```python
from build123d import *

# Parameters (mm, degrees)
SKETCH1_W                 = 77.5
SKETCH1_H                 = 31.5
BOSS_EXTRUDE1_DEPTH       = 2
CUT_EXTRUDE1_DEPTH        = 42.87630595
CUT_EXTRUDE1_DEPTH_BACK   = 42.87630595
SKETCH2_R                 = 1.75
CUT_EXTRUDE2_DEPTH        = 42.87630595
CUT_EXTRUDE2_DEPTH_BACK   = 42.87630595
SKETCH3_W                 = 8.5
SKETCH3_H                 = 15
BOSS_EXTRUDE2_START       = 3
SKETCH4_R                 = 2.5
SKETCH4_R_2               = 1.75
BOSS_EXTRUDE2_DEPTH       = 3
MIRROR2_START             = 3
MIRROR2_COPY_1_SKETCH_R   = 2.5
MIRROR2_COPY_1_SKETCH_R_2 = 1.75
MIRROR2_COPY_1_DEPTH      = 3
CUT_EXTRUDE3_DEPTH        = 3.5
SKETCH6_W                 = 8
SKETCH6_H                 = 10
SKETCH6_W_2               = 5
SKETCH6_H_2               = 4
BOSS_EXTRUDE3_DEPTH       = 3
SKETCH7_W                 = 16
SKETCH7_H                 = 7.5
BOSS_EXTRUDE4_DEPTH       = 3
CUT_EXTRUDE4_DEPTH        = 1
FILLET1_R                 = 10
FILLET2_R                 = 10
SKETCH9_R                 = 4
BOSS_EXTRUDE6_DEPTH       = 1.5


with BuildPart() as part:
    # Sketch1 → Boss-Extrude1 (new body)
    with BuildSketch(Plane(origin=(0, 0, 0), x_dir=(1, 0, 0), z_dir=(0, 1, 0))):
        Rectangle(SKETCH1_W, SKETCH1_H)
    extrude(amount=BOSS_EXTRUDE1_DEPTH)

    # Sketch2 → Cut-Extrude1 (cut, two sides: drawn at the far end of the back side and taken through both)
    with BuildSketch(Plane(origin=(0, 2, 0), x_dir=(1, 0, 0), z_dir=(0, 1, 0)).offset(-CUT_EXTRUDE1_DEPTH_BACK)):
        with Locations(Location((-35.75, 12.5, 0), (0, 0, 270))):
            Circle(SKETCH2_R)
        with Locations(Location((-35.75, -12.5, 0), (0, 0, 270))):
            Circle(SKETCH2_R)
        with Locations(Location((35.75, -12.5, 0), (0, 0, 270))):
            Circle(SKETCH2_R)
        with Locations(Location((35.75, 12.5, 0), (0, 0, 270))):
            Circle(SKETCH2_R)
    extrude(amount=CUT_EXTRUDE1_DEPTH + CUT_EXTRUDE1_DEPTH_BACK, mode=Mode.SUBTRACT)

    # Sketch3 → Cut-Extrude2 (cut, two sides: drawn at the far end of the back side and taken through both)
    with BuildSketch(Plane(origin=(0, 2, 0), x_dir=(1, 0, 0), z_dir=(0, 1, 0)).offset(-CUT_EXTRUDE2_DEPTH_BACK)):
        with Locations((31.5, 0)):
            Rectangle(SKETCH3_W, SKETCH3_H)
        with Locations((-31.5, 0)):
            Rectangle(SKETCH3_W, SKETCH3_H)
    extrude(amount=CUT_EXTRUDE2_DEPTH + CUT_EXTRUDE2_DEPTH_BACK, mode=Mode.SUBTRACT)

    # Sketch4 → Boss-Extrude2 (add)
    with BuildSketch(Plane(origin=(0, 2, 0), x_dir=(1, 0, 0), z_dir=(0, 1, 0)).offset(BOSS_EXTRUDE2_START)):
        with Locations(Location((-35.75, 12.5, 0), (0, 0, 270))):
            Circle(SKETCH4_R)
        with Locations(Location((-35.75, 12.5, 0), (0, 0, 270))):
            Circle(SKETCH4_R_2, mode=Mode.SUBTRACT)
    boss_extrude2 = extrude(amount=-BOSS_EXTRUDE2_DEPTH)

    # Mirror1: Boss-Extrude2 across plane
    add(boss_extrude2.mirror(Plane.XY))

    # Mirror2: Boss-Extrude2 across plane
    add(boss_extrude2.mirror(Plane(origin=(0, 0, 0), x_dir=(0, 0, 1), z_dir=(1, 0, 0))))

    # Mirror2 copy 1 sketch → Mirror2 copy 1 (add)
    with BuildSketch(Plane(origin=(0, 2, 0), x_dir=(-1, 0, 0), z_dir=(0, 1, 0)).offset(MIRROR2_START)):
        with Locations(Location((-35.75, 12.5, 0), (0, 0, 270))):
            Circle(MIRROR2_COPY_1_SKETCH_R)
        with Locations(Location((-35.75, 12.5, 0), (0, 0, 270))):
            Circle(MIRROR2_COPY_1_SKETCH_R_2, mode=Mode.SUBTRACT)
    extrude(amount=-MIRROR2_COPY_1_DEPTH)

    # Sketch5 → Cut-Extrude3 (cut)
    with BuildSketch(Plane(origin=(0, 2, 0), x_dir=(1, 0, 0), z_dir=(0, 1, 0))):
        with BuildLine():
            Line((19.75, -4.75), (19.75, 3.25))
            Line((19.75, 3.25), (20.25, 3.25))
            Line((20.25, 3.25), (20.25, -4.75))
            ThreePointArc((20.25, -4.75), (14.75, -10.25), (9.25, -4.75))
            Line((9.25, -4.75), (9.25, 3.25))
            Line((9.25, 3.25), (9.75, 3.25))
            Line((9.75, 3.25), (9.75, -4.75))
            ThreePointArc((9.75, -4.75), (14.75, -9.75), (19.75, -4.75))
        make_face()
        with BuildLine():
            Line((-19.75, 3.25), (-20.25, 3.25))
            Line((-20.25, 3.25), (-20.25, -4.75))
            ThreePointArc((-20.25, -4.75), (-14.75, -10.25), (-9.25, -4.75))
            Line((-9.25, -4.75), (-9.25, 3.25))
            Line((-9.25, 3.25), (-9.75, 3.25))
            Line((-9.75, 3.25), (-9.75, -4.75))
            ThreePointArc((-9.75, -4.75), (-14.75, -9.75), (-19.75, -4.75))
            Line((-19.75, -4.75), (-19.75, 3.25))
        make_face()
    extrude(amount=-CUT_EXTRUDE3_DEPTH, mode=Mode.SUBTRACT)

    # Sketch6 → Boss-Extrude3 (add)
    with BuildSketch(Plane(origin=(0, 2, 0), x_dir=(1, 0, 0), z_dir=(0, 1, 0))):
        with Locations((0, -2.75)):
            Rectangle(SKETCH6_W, SKETCH6_H)
        with Locations((5.5, 11.75)):
            Rectangle(SKETCH6_W_2, SKETCH6_H_2)
        with Locations((17.5, 11.75)):
            Rectangle(SKETCH6_W_2, SKETCH6_H_2)
        with Locations((-17.5, 11.75)):
            Rectangle(SKETCH6_W_2, SKETCH6_H_2)
        with Locations((-5.5, 11.75)):
            Rectangle(SKETCH6_W_2, SKETCH6_H_2)
    extrude(amount=BOSS_EXTRUDE3_DEPTH)

    # Sketch7 → Boss-Extrude4 (add)
    with BuildSketch(Plane(origin=(0, 2, 0), x_dir=(1, 0, 0), z_dir=(0, 1, 0))):
        with Locations((0, 6)):
            Rectangle(SKETCH7_W, SKETCH7_H)
    extrude(amount=BOSS_EXTRUDE4_DEPTH)

    # Sketch8 → Cut-Extrude4 (cut)
    with BuildSketch(Plane(origin=(0, 2, 0), x_dir=(1, 0, 0), z_dir=(0, 1, 0))):
        with BuildLine():
            Line((-9.75, 3.25), (-9.75, -4.75))
            ThreePointArc((-9.75, -4.75), (-14.75, -9.75), (-19.75, -4.75))
            Line((-19.75, -4.75), (-19.75, 3.25))
            Line((-19.75, 3.25), (-9.75, 3.25))
        make_face()
        with BuildLine():
            Line((19.75, 3.25), (9.75, 3.25))
            Line((9.75, 3.25), (9.75, -4.75))
            ThreePointArc((9.75, -4.75), (14.75, -9.75), (19.75, -4.75))
            Line((19.75, -4.75), (19.75, 3.25))
        make_face()
    extrude(amount=-CUT_EXTRUDE4_DEPTH, mode=Mode.SUBTRACT)

    # Fillet1
    # the kernel refuses this fillet: 10 mm, written as the material it takes off along each edge
    with BuildSketch(Plane(origin=(-4.75, 2, -3.25), x_dir=(0, 0, -1), z_dir=(-1, 0, 0))) as fillet1_piece_1_section:
        with BuildLine():
            CenterArc((6, 10), FILLET1_R, 233.130102354, 36.869897646)
            Line((0, 2), (0, 0))
            Line((0, 0), (6, 0))
        make_face()
    fillet1_piece_1 = extrude(amount=15.5, mode=Mode.PRIVATE)
    fillet1_piece_1 = split(fillet1_piece_1, bisect_by=Plane(origin=(-9.25, 2, -3.25), z_dir=(-1, 0, 0)), keep=Keep.TOP, mode=Mode.PRIVATE)
    fillet1_piece_1 = split(fillet1_piece_1, bisect_by=Plane(origin=(-4.75, 1, -3.25), z_dir=(0, 1, 0)), keep=Keep.TOP, mode=Mode.PRIVATE)
    add(fillet1_piece_1, mode=Mode.SUBTRACT)
    with BuildSketch(Plane(origin=(-4.75, 2, -3.25), x_dir=(0, 0, -1), z_dir=(-1, 0, 0))) as fillet1_piece_2_section:
        with BuildLine():
            CenterArc((6, 10), FILLET1_R, 233.130102354, 36.869897646)
            Line((0, 2), (0, 0))
            Line((0, 0), (6, 0))
        make_face()
    fillet1_piece_2 = extrude(amount=30.5, mode=Mode.PRIVATE)
    fillet1_piece_2 = split(fillet1_piece_2, bisect_by=Plane(origin=(-9.25, 2, -3.25), z_dir=(-1, 0, 0)), keep=Keep.TOP, mode=Mode.PRIVATE)
    fillet1_piece_2 = split(fillet1_piece_2, bisect_by=Plane(origin=(-9.75, 2, -3.25), z_dir=(1, 0, 0)), keep=Keep.TOP, mode=Mode.PRIVATE)
    add(fillet1_piece_2, mode=Mode.SUBTRACT)
    with BuildSketch(Plane(origin=(-19.75, 2, -3.25), x_dir=(0, 0, -1), z_dir=(-1, 0, 0)), Plane(origin=(-9.25, 2, -3.25), x_dir=(0, 0, -1), z_dir=(-1, 0, 0))) as fillet1_piece_3:
        with BuildLine():
            CenterArc((6, 10), FILLET1_R, 233.130102354, 36.869897646)
            Line((0, 2), (0, 0))
            Line((0, 0), (6, 0))
        make_face()
    extrude(amount=0.5, mode=Mode.SUBTRACT)
    with BuildSketch(Plane(origin=(-9.25, 2, -3.25), x_dir=(0, 0, -1), z_dir=(-1, 0, 0))) as fillet1_piece_4_section:
        with BuildLine():
            CenterArc((6, 10), FILLET1_R, 233.130102354, 36.869897646)
            Line((0, 2), (0, 0))
            Line((0, 0), (6, 0))
        make_face()
    fillet1_piece_4 = extrude(amount=15.5, mode=Mode.PRIVATE)
    fillet1_piece_4 = split(fillet1_piece_4, bisect_by=Plane(origin=(-20.25, 2, -3.25), z_dir=(1, 0, 0)), keep=Keep.TOP, mode=Mode.PRIVATE)
    fillet1_piece_4 = split(fillet1_piece_4, bisect_by=Plane(origin=(-9.25, 1, -3.25), z_dir=(0, 1, 0)), keep=Keep.TOP, mode=Mode.PRIVATE)
    add(fillet1_piece_4, mode=Mode.SUBTRACT)
    with BuildSketch(Plane(origin=(5.75, 2, -3.25), x_dir=(0, 0, -1), z_dir=(-1, 0, 0))) as fillet1_piece_5_section:
        with BuildLine():
            CenterArc((6, 10), FILLET1_R, 233.130102354, 36.869897646)
            Line((0, 2), (0, 0))
            Line((0, 0), (6, 0))
        make_face()
    fillet1_piece_5 = extrude(amount=30.5, mode=Mode.PRIVATE)
    fillet1_piece_5 = split(fillet1_piece_5, bisect_by=Plane(origin=(-20.25, 2, -3.25), z_dir=(1, 0, 0)), keep=Keep.TOP, mode=Mode.PRIVATE)
    fillet1_piece_5 = split(fillet1_piece_5, bisect_by=Plane(origin=(-19.75, 2, -3.25), z_dir=(-1, 0, 0)), keep=Keep.TOP, mode=Mode.PRIVATE)
    add(fillet1_piece_5, mode=Mode.SUBTRACT)
    with BuildSketch(Plane(origin=(4.75, 2, -3.25), x_dir=(0, 0, -1), z_dir=(1, 0, 0))) as fillet1_piece_6_section:
        with BuildLine():
            CenterArc((6, -10), FILLET1_R, 90, 36.869897646)
            Line((0, -2), (0, 0))
            Line((0, 0), (6, 0))
        make_face()
    fillet1_piece_6 = extrude(amount=15.5, mode=Mode.PRIVATE)
    fillet1_piece_6 = split(fillet1_piece_6, bisect_by=Plane(origin=(9.25, 2, -3.25), z_dir=(1, 0, 0)), keep=Keep.TOP, mode=Mode.PRIVATE)
    fillet1_piece_6 = split(fillet1_piece_6, bisect_by=Plane(origin=(4.75, 1, -3.25), z_dir=(0, 1, 0)), keep=Keep.TOP, mode=Mode.PRIVATE)
    add(fillet1_piece_6, mode=Mode.SUBTRACT)
    with BuildSketch(Plane(origin=(4.75, 2, -3.25), x_dir=(0, 0, -1), z_dir=(1, 0, 0))) as fillet1_piece_7_section:
        with BuildLine():
            CenterArc((6, -10), FILLET1_R, 90, 36.869897646)
            Line((0, -2), (0, 0))
            Line((0, 0), (6, 0))
        make_face()
    fillet1_piece_7 = extrude(amount=30.5, mode=Mode.PRIVATE)
    fillet1_piece_7 = split(fillet1_piece_7, bisect_by=Plane(origin=(9.75, 2, -3.25), z_dir=(-1, 0, 0)), keep=Keep.TOP, mode=Mode.PRIVATE)
    fillet1_piece_7 = split(fillet1_piece_7, bisect_by=Plane(origin=(9.25, 2, -3.25), z_dir=(1, 0, 0)), keep=Keep.TOP, mode=Mode.PRIVATE)
    add(fillet1_piece_7, mode=Mode.SUBTRACT)
    with BuildSketch(Plane(origin=(19.75, 2, -3.25), x_dir=(0, 0, -1), z_dir=(1, 0, 0)), Plane(origin=(9.25, 2, -3.25), x_dir=(0, 0, -1), z_dir=(1, 0, 0))) as fillet1_piece_8:
        with BuildLine():
            CenterArc((6, -10), FILLET1_R, 90, 36.869897646)
            Line((0, -2), (0, 0))
            Line((0, 0), (6, 0))
        make_face()
    extrude(amount=0.5, mode=Mode.SUBTRACT)
    with BuildSketch(Plane(origin=(9.25, 2, -3.25), x_dir=(0, 0, -1), z_dir=(1, 0, 0))) as fillet1_piece_9_section:
        with BuildLine():
            CenterArc((6, -10), FILLET1_R, 90, 36.869897646)
            Line((0, -2), (0, 0))
            Line((0, 0), (6, 0))
        make_face()
    fillet1_piece_9 = extrude(amount=15.5, mode=Mode.PRIVATE)
    fillet1_piece_9 = split(fillet1_piece_9, bisect_by=Plane(origin=(20.25, 2, -3.25), z_dir=(-1, 0, 0)), keep=Keep.TOP, mode=Mode.PRIVATE)
    fillet1_piece_9 = split(fillet1_piece_9, bisect_by=Plane(origin=(9.25, 1, -3.25), z_dir=(0, 1, 0)), keep=Keep.TOP, mode=Mode.PRIVATE)
    add(fillet1_piece_9, mode=Mode.SUBTRACT)
    with BuildSketch(Plane(origin=(-5.75, 2, -3.25), x_dir=(0, 0, -1), z_dir=(1, 0, 0))) as fillet1_piece_10_section:
        with BuildLine():
            CenterArc((6, -10), FILLET1_R, 90, 36.869897646)
            Line((0, -2), (0, 0))
            Line((0, 0), (6, 0))
        make_face()
    fillet1_piece_10 = extrude(amount=30.5, mode=Mode.PRIVATE)
    fillet1_piece_10 = split(fillet1_piece_10, bisect_by=Plane(origin=(19.75, 2, -3.25), z_dir=(1, 0, 0)), keep=Keep.TOP, mode=Mode.PRIVATE)
    fillet1_piece_10 = split(fillet1_piece_10, bisect_by=Plane(origin=(20.25, 2, -3.25), z_dir=(-1, 0, 0)), keep=Keep.TOP, mode=Mode.PRIVATE)
    add(fillet1_piece_10, mode=Mode.SUBTRACT)

    # Fillet2
    # the kernel refuses this fillet: 10 mm, written as the material it adds along each edge
    with BuildSketch(Plane(origin=(19.75, 1, -4.891101056), x_dir=(0, 0.3749043717325089, -0.9270634886866448), z_dir=(-1, 0, 0))) as fillet2_piece_1:
        with BuildLine():
            CenterArc((2.000510148, -9.977741668), FILLET2_R, 93.823530212, 18.194872339)
            Line((-1.74853357, -0.707106781), (0, 0))
            ThreePointArc((0, 0), (0.666836716, -0.022258332), (1.333673432, 0))
        make_face()
    extrude(amount=10)
    with BuildSketch(Plane(origin=(-19.75, 1, -4.891101056), x_dir=(0, 0.3749043717325089, -0.9270634886866448), z_dir=(1, 0, 0))) as fillet2_piece_2:
        with BuildLine():
            CenterArc((2.000510148, 9.977741668), FILLET2_R, 247.981597449, 18.194872339)
            Line((-1.74853357, 0.707106781), (0, 0))
            ThreePointArc((0, 0), (0.666836716, 0.022258332), (1.333673432, 0))
        make_face()
    extrude(amount=10)

    # Sketch9 → Boss-Extrude6 (add)
    with BuildSketch(Plane(origin=(0, 1, 0), x_dir=(1, 0, 0), z_dir=(0, 1, 0))):
        with Locations(Location((14.75, -4.75, 0), (0, 0, 90))):
            Circle(SKETCH9_R)
        with Locations(Location((-14.75, -4.75, 0), (0, 0, 90))):
            Circle(SKETCH9_R)
    extrude(amount=BOSS_EXTRUDE6_DEPTH)


solid = part.part
```
Part model, mm, in its own coordinate system. A direction names the side the tool comes from. Round coordinates to 2 decimals unless told otherwise and drop trailing zeros. Write each loop counter-clockwise with the first axis right and the second up, starting at its lowest first coordinate (ties: lowest second). Pieces come first, ordered by that corner, then holes. Notation, with made-up numbers: M -19.75,-1.5 L -1.75,-1.5 A29 cw -1.75,19.5 Z; hole C 60.25,58.25 d11. An arc over 180 degrees is marked long. Answer as CSV lines item,"result". Start each with the question number.
1) Mould opens along X. For faces 1 (the face through (-37, 5, -11)), 2 (the face through (3, 3, -12)), 3 (the face through (15, 3, -12)), 4 (the face through (38.75, 1, 0)) say: +X half, -X half, draft (parallel to the pull), parting line (faces both ways), or undercut.
2) Band-saw the part on C-C (x = 6.5). List the corners of the cut face in (y, z), then the cut area to 3 significant figures.
3) Drill centre lines: L1, parallel to X at y = 1.65, z = -5; L2, parallel to Z at x = 35.75, y = 3; L3, parallel to X at y = 0.5, z = -12.5. Where is each one in solid material? Low to high.
4) Which spindle directions (+Z, -Z, +X, -X, +Y, -Y) get a long thin tool onto all of the face, cutting with end or side? Do faces 5 (the face through (14.87, 1.01, 10.25)), 6 (the face through (-6, 3, -2.25)), 7 (the face through (34.06, 3.52, 14.34)). Say none if no direction does.
5) Band-saw the part on A-A (y = 3.3). Count the separate pieces of the cut face and the enclosed holes in it, then the cut area to 3 significant figures.
6) Drop flat-ended pins along their axis: pin 1 (2.5 mm diameter, centred on y = 3.5, z = -11.5, fed in from +X); pin 2 (11 mm diameter, centred on x = 16.5, z = 0.5, fed in from +Y); pin 3 (0.9 mm diameter, centred on x = -18.5, y = 3.5, fed in from +Z). Give the stop position or say it passes through.
7) Band-saw the part on B-B (z = 12.5). List the corners of the cut face in (x, y), then the cut area to 3 significant figures.
Worked out:
1,face 1,"draft"
1,face 2,"undercut"
1,face 3,"undercut"
1,face 4,"+X half"
2,outline,"M 0,-15.75 L 2,-15.75 L 2,-13.75 L 5,-13.75 L 5,-2.25 L 2,-2.25 L 2,15.75 L 0,15.75 Z"
2,area,"97.5 mm²"
3,L1,"-38.75 to -35.75, -27.25 to -20.25, -9.25 to 9.25, 20.25 to 27.25, 35.75 to 38.75"
3,L2,"-15 to -14.25, -10.75 to -10, 10 to 10.75, 14.25 to 15"
3,L3,"-38.75 to -37.5, -34 to 34, 37.5 to 38.75"
4,face 5,"+Y, -Y"
4,face 6,"+Z, -X, +Y"
4,face 7,"+Y"
5,separate pieces,"7"
5,enclosed holes,"4"
5,area,"320 mm²"
6,pin 1,"x = 38.25"
6,pin 2,"y = 2.5"
6,pin 3,"z = -9.75"
7,outline,"M -38.75,0 L -37.5,0 L -37.5,5 L -38.25,5 L -38.25,2 L -38.75,2 Z; M -34,0 L 34,0 L 34,5 L 33.25,5 L 33.25,2 L -33.25,2 L -33.25,5 L -34,5 Z; M 37.5,0 L 38.75,0 L 38.75,2 L 38.25,2 L 38.25,5 L 37.5,5 Z"
7,area,"150 mm²"
